CAD build for the part. Positions are in the model's coordinates, mm. Round coordinates to 2 decimals unless told otherwise and drop trailing zeros. Loops run counter-clockwise (first coordinate to the right, second up) from the corner with the lowest first, then second, coordinate; pieces in that order, holes last. Notation, with made-up numbers: M 8,-5.5 L 50,-5.5 A16 cw 50,9.5 Z; hole C -8.75,-36.75 d3. An arc over 180 degrees is marked long. One line per item, written item: value. Start each with the question number.
from build123d import *

# Parameters (mm, degrees)
BOSS_EXTRUDE1_DEPTH = 5


with BuildPart() as part:
    # Sketch1 → Boss-Extrude1 (new body, symmetric)
    with BuildSketch(Plane.XY):
        with BuildLine():
            Line((175, 125), (175, -125))
            Line((175, -125), (125, -175))
            Line((125, -175), (50, -175))
            ThreePointArc((50, -175), (0, -125), (-50, -175))
            Line((-50, -175), (-125, -175))
            Line((-125, -175), (-175, -125))
            Line((-175, -125), (-175, 125))
            Line((-175, 125), (-125, 175))
            Line((-125, 175), (-50, 175))
            ThreePointArc((-50, 175), (0, 125), (50, 175))
            Line((50, 175), (125, 175))
            Line((125, 175), (175, 125))
        make_face()
    extrude(amount=BOSS_EXTRUDE1_DEPTH, both=True)


solid = part.part
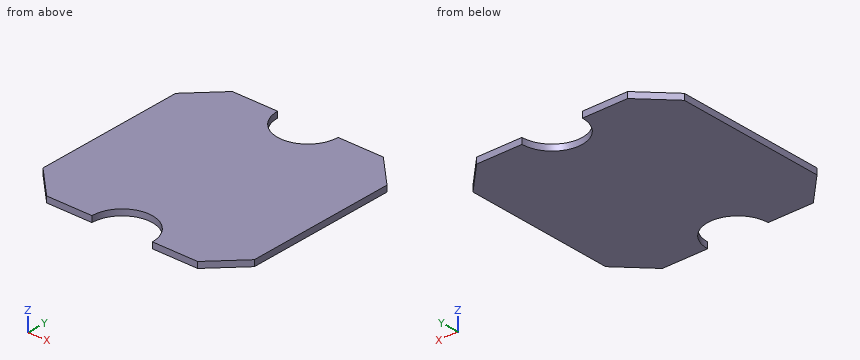
(1) Slice it at B-B, the plane z = 2. List the corners of the cut face in (x, y), and give its area (3 significant figures).
(2) Flat gauge pins, fed straight in: P1, Ø4, axis at y = -139, z = -0.5, coming from the +X side; P2, Ø4, axis at x = -33.5, z = -1, coming from the -Y side. Where does each tip first touch, or does it go through?
(3) Slice it at A-A, the plane y = -144.5. List the corners of the cut face in (x, z), and give its area (3 significant figures).
(4) Probe L1, parallel to X at y = -149, z = 1; L2, parallel to X at y = -146.5, z = -3.25; L3, parallel to Y at x = 134.5, z = 1. List the from-to ranges inside material, lowest first.
(5) Slice it at C-C, the plane x = 0. List the corners of the cut face in (y, z), and give its area (3 significant figures).
Check result:
1. outline: M -175,-125 L -125,-175 L -50,-175 A50 cw 50,-175 L 125,-175 L 175,-125 L 175,125 L 125,175 L 50,175 A50 cw -50,175 L -125,175 L -175,125 Z
1. area: 110,000 mm^2
2. P1: stops at x = 163
2. P2: stops at y = -139.79
3. outline: M -155.5,-5 L -39.62,-5 L -39.62,5 L -155.5,5 Z; M 39.62,-5 L 155.5,-5 L 155.5,5 L 39.62,5 Z
3. area: 2,320 mm^2
4. L1: x = -151 to -42.71, 42.71 to 151
4. L2: x = -153.5 to -41.08, 41.08 to 153.5
4. L3: y = -165.5 to 165.5
5. outline: M -125,-5 L 125,-5 L 125,5 L -125,5 Z
5. area: 2,500 mm^2
